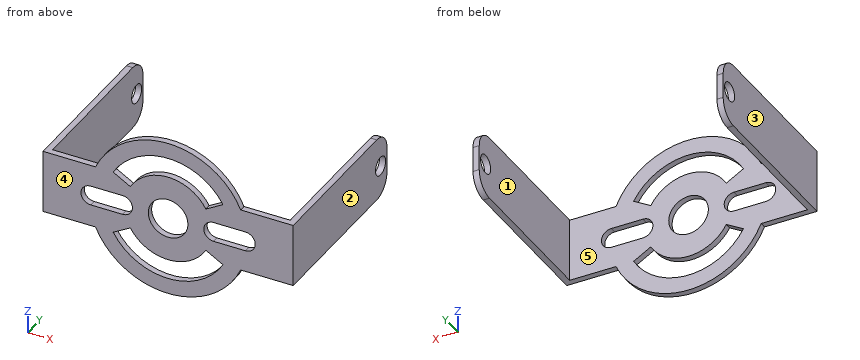
```python
from build123d import *

# Parameters (mm, degrees)
SKETCH1_R           = 3.175
BOSS_EXTRUDE1_DEPTH = 1
BOSS_EXTRUDE2_DEPTH = 1
BOSS_EXTRUDE3_START = 1
BOSS_EXTRUDE3_DEPTH = 1
SKETCH4_R           = 1.5
CUT_EXTRUDE1_DEPTH  = 51.4944901


with BuildPart() as part:
    # Sketch1 → Boss-Extrude1 (new body)
    with BuildSketch(Plane(origin=(0, 0, 0), x_dir=(1, 0, 0), z_dir=(0, 1, 0))):
        with BuildLine():
            Line((11.628995247, 5.08), (19.05, 5.08))
            Line((19.05, 5.08), (19.05, -5.08))
            Line((19.05, -5.08), (11.628995247, -5.08))
            ThreePointArc((11.628995247, -5.08), (0, -12.690150923), (-11.628995247, -5.08))
            Line((-11.628995247, -5.08), (-19.05, -5.08))
            Line((-19.05, -5.08), (-19.05, 5.08))
            Line((-19.05, 5.08), (-11.628995247, 5.08))
            ThreePointArc((-11.628995247, 5.08), (0, 12.690150923), (11.628995247, 5.08))
        make_face()
        with Locations(Location((0, 0, 0), (0, 0, 270))):
            Circle(SKETCH1_R, mode=Mode.SUBTRACT)
        with BuildLine():
            Line((8.798818102, 5.08), (6.049187445, 3.4925))
            ThreePointArc((6.049187445, 3.4925), (0, 6.983078605), (-6.049187445, 3.4925))
            Line((-6.049187445, 3.4925), (-8.798818102, 5.08))
            ThreePointArc((-8.798818102, 5.08), (0, 10.158078357), (8.798818102, 5.08))
        make_face(mode=Mode.SUBTRACT)
        with BuildLine():
            Line((8.798818102, -5.08), (6.049187445, -3.4925))
            ThreePointArc((6.049187445, -3.4925), (0, -6.986922982), (-6.049187445, -3.4925))
            Line((-6.049187445, -3.4925), (-8.798818102, -5.08))
            ThreePointArc((-8.798818102, -5.08), (0, -10.161922734), (8.798818102, -5.08))
        make_face(mode=Mode.SUBTRACT)
        with BuildLine():
            Line((12.3825, -1.5875), (7.3025, -1.5875))
            ThreePointArc((7.3025, -1.5875), (5.715, 0), (7.3025, 1.5875))
            Line((7.3025, 1.5875), (12.3825, 1.5875))
            ThreePointArc((12.3825, 1.5875), (13.97, 0), (12.3825, -1.5875))
        make_face(mode=Mode.SUBTRACT)
        with BuildLine():
            Line((-7.3025, 1.5875), (-12.3825, 1.5875))
            ThreePointArc((-12.3825, 1.5875), (-13.97, 0), (-12.3825, -1.5875))
            Line((-12.3825, -1.5875), (-7.3025, -1.5875))
            ThreePointArc((-7.3025, -1.5875), (-5.715, 0), (-7.3025, 1.5875))
        make_face(mode=Mode.SUBTRACT)
    extrude(amount=BOSS_EXTRUDE1_DEPTH)

    # Sketch2 → Boss-Extrude2 (add)
    with BuildSketch(Plane(origin=(19.05, 0, -13.97), x_dir=(0, 0, -1), z_dir=(1, 0, 0))):
        with BuildLine():
            Line((-19.05, 0), (-8.89, 0))
            Line((-8.89, 0), (-8.89, 24.892))
            ThreePointArc((-8.89, 24.892), (-9.782738531, 27.047261469), (-11.938, 27.94))
            Line((-11.938, 27.94), (-16.002, 27.94))
            ThreePointArc((-16.002, 27.94), (-18.157261469, 27.047261469), (-19.05, 24.892))
            Line((-19.05, 24.892), (-19.05, 0))
        make_face()
    extrude(amount=BOSS_EXTRUDE2_DEPTH)

    # Sketch3 → Boss-Extrude3 (add)
    with BuildSketch(Plane(origin=(-19.05, 0, 13.97), x_dir=(0, 0, 1), z_dir=(-1, 0, 0)).offset(BOSS_EXTRUDE3_START)):
        with BuildLine():
            Line((-8.89, 0), (-19.05, 0))
            Line((-19.05, 0), (-19.05, 24.892))
            ThreePointArc((-19.05, 24.892), (-18.157261469, 27.047261469), (-16.002, 27.94))
            Line((-16.002, 27.94), (-11.938, 27.94))
            ThreePointArc((-11.938, 27.94), (-9.782738531, 27.047261469), (-8.89, 24.892))
            Line((-8.89, 24.892), (-8.89, 0))
        make_face()
    extrude(amount=-BOSS_EXTRUDE3_DEPTH)

    # Sketch4 → Cut-Extrude1 (cut, through all)
    with BuildSketch(Plane.ZY.offset(20.05)):
        with Locations((0, 26.035)):
            Circle(SKETCH4_R)
    extrude(amount=-CUT_EXTRUDE1_DEPTH, mode=Mode.SUBTRACT)


solid = part.part
```
Design review of the part built by this model. Coordinates are the model's own, in mm. Face numbers are marked on the shaded views. A direction names the side the tool comes from. Round coordinates to 2 decimals unless told otherwise and drop trailing zeros. Order: outer loops, then holes, each group sorted by start corner. A loop starts at its lowest first (then second) coordinate and runs counter-clockwise, first axis right, second up. Notation, with made-up numbers: M 17.5,56.5 L 72.5,56.5 A7 cw 72.5,66.5 Z; hole C 6,4 d4. An arc over 180 degrees is marked long. Put each result on its own line as item: value.
Q1. Consider section B-B (x = 0). State the section outline as (y, z) points (3 decimals).
Reported:
outline: M 0,-12.69 L 1,-12.69 L 1,-10.158 L 0,-10.158 Z; M 0,-6.983 L 1,-6.983 L 1,-3.175 L 0,-3.175 Z; M 0,3.175 L 1,3.175 L 1,6.987 L 0,6.987 Z; M 0,10.162 L 1,10.162 L 1,12.69 L 0,12.69 Z
Q2. Insertion check: pin 1 Ø3.5 at (y, z) = (26.035, 0) entering from +X; pin 2 Ø6.5 at (x, y) = (-16, 8.5) entering from -Z; pin 3 Ø2 at (x, z) = (13, 6) entering from +Y; pin 4 Ø12 at (x, y) = (10, 23) entering from +Z. Each pin has a flat end and moves straight along its axis. Give the tip position at first contact, or say it passes through.
Reported:
pin 1: x = 20.05
pin 2: z = -5.08
pin 3: y = 1
pin 4: through
Q3. To check wall thickness, follow line 1 (X direction, y = 0.5, z = 0) (3 decimals); line 2 (X direction, y = 3.5, z = 0.25); line 3 (Y direction, x = 19.8, z = 0) (3 decimals). State the ranges of each line that lie inside material, in increasing order.
Reported:
line 1: -20.05 to -13.97, -5.715 to -3.175, 3.175 to 5.715, 13.97 to 20.05
line 2: -20.05 to -19.05, 19.05 to 20.05
line 3: 0 to 24.535, 27.535 to 27.94
Q4. Consider section D-D (z = 6.25). State the section outline as (x, y) points.
Reported:
outline: M -11.04,0 L -8.01,0 L -8.01,1 L -11.04,1 Z; M -3.12,0 L 3.12,0 L 3.12,1 L -3.12,1 Z; M 8.01,0 L 11.04,0 L 11.04,1 L 8.01,1 Z
Q5. Consider section C-C (z = 0). State the section outline as (x, y) points (3 decimals), and give its area (3 significant figures).
Reported:
outline: M -20.05,0 L -13.97,0 L -13.97,1 L -19.05,1 L -19.05,24.535 L -20.05,24.535 Z; M -20.05,27.535 L -19.05,27.535 L -19.05,27.94 L -20.05,27.94 Z; M -5.715,0 L -3.175,0 L -3.175,1 L -5.715,1 Z; M 3.175,0 L 5.715,0 L 5.715,1 L 3.175,1 Z; M 13.97,0 L 20.05,0 L 20.05,24.535 L 19.05,24.535 L 19.05,1 L 13.97,1 Z; M 19.05,27.535 L 20.05,27.535 L 20.05,27.94 L 19.05,27.94 Z
area: 65.1 mm²
Q6. Machinability: for the marked faces 4 and 5, which of the approach directions +Z, -Z, +X, -X, +Y, -Y give a long, thin tool a straight path to every point of the face, cutting with its end or side? Answer none if there is none.
Reported:
face 4: +Z, -Z, +X, -X, -Y
face 5: +Z, -Z, +Y
Q7. Draft analysis for pull direction X (two halves, no side actions). For the marked faces 1, 2 and 3, state which applies: released by +X, released by -X, zero draft, split by the parting line, or undercut.
Reported:
face 1: undercut
face 2: released by +X
face 3: released by -X
Q8. Consider section A-A (y = 14.25). State the section outline as (x, z) points, and give its area (3 significant figures).
Reported:
outline: M -20.05,-5.08 L -19.05,-5.08 L -19.05,5.08 L -20.05,5.08 Z; M 19.05,-5.08 L 20.05,-5.08 L 20.05,5.08 L 19.05,5.08 Z
area: 20.3 mm²
